Verification items for the finished model (mm, model axes). Coordinates: 2 decimals unless noted, no trailing zeros. Loops run counter-clockwise (first coordinate to the right, second up) from the corner with the lowest first, then second, coordinate; pieces in that order, holes last.
Q1. Sectioned sample at A-A (y = 55.5). Enter the section's corners in (x, z).
Q2. Mould release check, pull along Z, two halves, no side actions. Record for faces 1 (the face through (-1.38, 129.17, 6.2)), 2 (the face through (0, 0, 0)): +Z half, -Z half, draft (parallel to the pull), parting line (faces both ways), or undercut.
Q3. Go/stop test with flat-tipped pins: P1, Ø5, axis at x = 4, y = 135.5, coming from the +Z side; P2, Ø1.8, axis at y = 127, z = -5.5, coming from the +X side; P3, Ø3, axis at y = 41, z = -4, coming from the +X side. Record where each tip stops, or that it passes through.
Q4. Material ranges on probe 1 along Z at (x, y) = (-0.5, 88); probe 2 along X at (y, z) = (199, 0.75); probe 3 along Z at (x, y) = (-2, 201), recorded low to high.
Q5. Sectioned sample at B-B (z = 2.25). Enter the section's corners in (x, y), then the cut area to 3 significant figures.
```python
from build123d import *

# Parameters (mm, degrees)
SKETCH1_R               = 6.35
BOSS_EXTRUDE1_DEPTH     = 262
SKETCH2_W               = 3.175
SKETCH2_H               = 3.2004
CUT_EXTRUDE1_DEPTH      = 12.7
CUT_EXTRUDE1_DEPTH_BACK = 12.7


with BuildPart() as part:
    # Sketch1 → Boss-Extrude1 (new body)
    with BuildSketch(Plane(origin=(0, 0, 0), x_dir=(1, 0, 0), z_dir=(0, 1, 0))):
        Circle(SKETCH1_R)
    extrude(amount=BOSS_EXTRUDE1_DEPTH)

    # Sketch2 → Cut-Extrude1 (cut, two sides)
    with BuildSketch(Plane(origin=(0, 131, 0), x_dir=(1, 0, 0), z_dir=(0, 1, 0))) as cut_extrude1_sk:
        with Locations((0, 6.148361062)):
            Rectangle(SKETCH2_W, SKETCH2_H)
    extrude(amount=CUT_EXTRUDE1_DEPTH, mode=Mode.SUBTRACT)
    extrude(cut_extrude1_sk.sketch, amount=-CUT_EXTRUDE1_DEPTH_BACK, mode=Mode.SUBTRACT)


solid = part.part
```
Geometry check:
1. outline: circle Ø12.7 at (0, 0)
2. face 1: parting line
2. face 2: draft
3. P1: stops at z = 6.17
3. P2: stops at x = 4.38
3. P3: stops at x = 5.84
4. probe 1: z = -6.33 to 6.33
4. probe 2: x = -6.31 to 6.31
4. probe 3: z = -6.03 to 6.03
5. outline: (-5.94, 0) - (5.94, 0) - (5.94, 262) - (-5.94, 262) - close
5. area: 3,110 mm2
